Verification items for the finished model (mm, model axes). A direction names the side the tool comes from. Round coordinates to 2 decimals unless told otherwise and drop trailing zeros. Order: outer loops, then holes, each group sorted by start corner. A loop starts at its lowest first (then second) coordinate and runs counter-clockwise, first axis right, second up. Notation, with made-up numbers: M 56,-30.5 L 81,-30.5 A16 ccw 81,-12.5 Z; hole C -9,65 d7. An arc over 180 degrees is marked long. Answer as a JSON object with one key per item and string values. Group by question number.
```python
from build123d import *

# Parameters (mm, degrees)
SKETCH2_W           = 80
SKETCH2_H           = 80
BOSS_EXTRUDE1_DEPTH = 3.175
SKETCH3_OUTSIDE_W   = 104.636
SKETCH3_OUTSIDE_H   = 104.636
CUT_EXTRUDE1_DEPTH  = 57.657573413
SKETCH4_W           = 3.175
SKETCH4_H           = 49.1
CUT_EXTRUDE2_DEPTH  = 57.657573413


with BuildPart() as part:
    # Sketch2 → Boss-Extrude1 (new body)
    with BuildSketch(Plane(origin=(0, 0, 0), x_dir=(0, 0, -1), z_dir=(1, 0, 0))):
        Rectangle(SKETCH2_W, SKETCH2_H)
    extrude(amount=BOSS_EXTRUDE1_DEPTH)

    # Sketch3 outside → Cut-Extrude1 (cut, through all)
    with BuildSketch(Plane(origin=(3.175, 0, 0), x_dir=(0, 0, -1), z_dir=(1, 0, 0))):
        Rectangle(SKETCH3_OUTSIDE_W, SKETCH3_OUTSIDE_H)
        Polygon((34.666666667, 36.825), (36.825, 36.825), (36.825, 31.915), (40, 31.915), (40, 27.005), (36.825, 27.005), (36.825, 22.095), (40, 22.095), (40, 17.185), (36.825, 17.185), (36.825, 12.275), (40, 12.275), (40, 7.365), (36.825, 7.365), (36.825, 2.455), (40, 2.455), (40, -2.455), (36.825, -2.455), (36.825, -7.365), (40, -7.365), (40, -12.275), (36.825, -12.275), (36.825, -17.185), (40, -17.185), (40, -22.095), (36.825, -22.095), (36.825, -27.005), (40, -27.005), (40, -31.915), (36.825, -31.915), (36.825, -36.825), (34.666666667, -36.825), (34.666666667, -40), (29.333333333, -40), (29.333333333, -36.825), (24, -36.825), (24, -40), (18.666666667, -40), (18.666666667, -36.825), (13.333333333, -36.825), (13.333333333, -40), (8, -40), (8, -36.825), (2.666666667, -36.825), (2.666666667, -40), (-2.666666667, -40), (-2.666666667, -36.825), (-8, -36.825), (-8, -40), (-13.333333333, -40), (-13.333333333, -36.825), (-18.666666667, -36.825), (-18.666666667, -40), (-24, -40), (-24, -36.825), (-29.333333333, -36.825), (-29.333333333, -40), (-34.666666667, -40), (-34.666666667, -36.825), (-36.825, -36.825), (-36.825, -31.915), (-40, -31.915), (-40, -27.005), (-36.825, -27.005), (-36.825, -22.095), (-40, -22.095), (-40, -17.185), (-36.825, -17.185), (-36.825, -12.275), (-40, -12.275), (-40, -7.365), (-36.825, -7.365), (-36.825, -2.455), (-40, -2.455), (-40, 2.455), (-36.825, 2.455), (-36.825, 7.365), (-40, 7.365), (-40, 12.275), (-36.825, 12.275), (-36.825, 17.185), (-40, 17.185), (-40, 22.095), (-36.825, 22.095), (-36.825, 27.005), (-40, 27.005), (-40, 31.915), (-36.825, 31.915), (-36.825, 36.825), (-34.666666667, 36.825), (-34.666666667, 40), (-29.333333333, 40), (-29.333333333, 36.825), (-24, 36.825), (-24, 40), (-18.666666667, 40), (-18.666666667, 36.825), (-13.333333333, 36.825), (-13.333333333, 40), (-8, 40), (-8, 36.825), (-2.666666667, 36.825), (-2.666666667, 40), (2.666666667, 40), (2.666666667, 36.825), (8, 36.825), (8, 40), (13.333333333, 40), (13.333333333, 36.825), (18.666666667, 36.825), (18.666666667, 40), (24, 40), (24, 36.825), (29.333333333, 36.825), (29.333333333, 40), (34.666666667, 40), align=None, mode=Mode.SUBTRACT)
    extrude(amount=-CUT_EXTRUDE1_DEPTH, mode=Mode.SUBTRACT)

    # Sketch4 → Cut-Extrude2 (cut, through all)
    with BuildSketch(Plane(origin=(3.175, 0, 0), x_dir=(0, 0, -1), z_dir=(1, 0, 0))):
        with Locations((38.4125, -12.275)):
            Rectangle(SKETCH4_W, SKETCH4_H)
    extrude(amount=-CUT_EXTRUDE2_DEPTH, mode=Mode.SUBTRACT)


solid = part.part
```
Q1. Cross-section at A-A, the plane y = -35. Record the cut outline in (x, z) (3 decimals), then the cut area to 3 significant figures.
Q2. Thickness scan on line 1 (Z direction, x = 2.55, y = 22.5) (3 decimals); line 2 (Z direction, x = 2.15, y = 0) (3 decimals). Record the ranges inside material, lowest first. Write a range as from..to.
Q3. Tool access check on faces 4 (the face through (2, 38, -18.667)), 5 (the face through (2, -9, -36.825)), 6 (the face through (2, -2.455, 38)), 7 (the face through (2, -38, 24)). Record the directions out of +Z, -Z, +X, -X, +Y, -Y that give a thin tool (end or side, any length) a straight path to the whole face; none if there is none.
Q4. Gauge pin test, flat ends, axial feed: pin 1 Ø0.6 at (x, z) = (1.5, -35.5) entering from -Y (3 decimals); pin 2 Ø1.6 at (x, z) = (1, 38.5) entering from -Y (3 decimals); pin 3 Ø1.6 at (x, z) = (1.5, 38.5) entering from +Y (3 decimals). Record the tip position at first contact, or that the pin passes through.
Q5. Release check for a two-part mould opening along Y. For faces 1 (the face through (2, 2.455, 38)), 2 (the face through (2, -38, 2.667)), 3 (the face through (2, 40, -32)) record: released by +Y, released by -Y, zero draft, split by the parting line, or undercut.
Conclusion:
{
 "1": {"outline": "M 0,-36.825 L 3.175,-36.825 L 3.175,36.825 L 0,36.825 Z", "area": "234 mm2"},
 "2": {"line 1": "-36.825..36.825", "line 2": "-36.825..40"},
 "3": {"face 4": "+X, -X, +Y", "face 5": "-Z, +X, -X, -Y", "face 6": "+Z, +X, -X", "face 7": "+X, -X, -Y"},
 "4": {"pin 1": "y = -36.825", "pin 2": "y = -31.915", "pin 3": "y = 31.915"},
 "5": {"face 1": "undercut", "face 2": "zero draft", "face 3": "released by +Y"}
}
